Autodesk Fusion 360 part; units mm, degrees
sketch "profile" plane through (0, 0, 0) normal (0, 0, 1) x (1, 0, 0)
  line L0 (0, 0) -> (0, 14)
  line L1 (21.6, 10.2) -> (19.6, 11.8)
  line L2 (19.6, 11.8) -> (21.8, 14)
  line L3 (21.8, 14) -> (25.6, 14)
  line L4 (4, 10.2) -> (6, 11.8)
  line L5 (6, 11.8) -> (3.8, 14)
  line L6 (3.8, 14) -> (0, 14)
  line L7 (4, 4) -> (21.6, 4)
  line L8 (4, 10.2) -> (4, 4)
  line L9 (21.6, 4) -> (21.6, 10.2)
  line L10 (0, 0) -> (25.6, 0)
  line L11 (25.6, 14) -> (25.6, 0)
  dimension "d74" = 3.8
  dimension "d75" = 3.8
  dimension "d76" = 4
  dimension "d80" = 17.6
  dimension "d84" = 4
  dimension "d85" = 14
  dimension "d86" = 14
  dimension "d87" = 3.8
  dimension "d88" = 6
  dimension "d89" = 4
  dimension "d90" = 25.8
  dimension "d117" = 6
  dimension "d118" = 3.8
  dimension "d119" = 1.6
  dimension "d120" = 1.6
extrude "Extrude2" add sketch "profile" along normal blind 130
move_body "Move1" bodies 1 to x (1, 0, 0) y (0, 0, 1) z (0, -1, 0) at (0, 6.5916, 6.5916)
hole "Hole4" at (25.6, -58.4084, 13.5916) direction (-1, 0, 0) diameter 2.529 depth 42 tip angle 180
fillet "Fillet5" radius 2 1 edges at (25.6, -58.4084, 20.5916)
fillet "Fillet6" radius 2 1 edges at (0, -58.4084, 20.5916)
fillet "Fillet7" radius 2 2 edges at (21.8, -58.4084, 20.5916) (3.8, -58.4084, 20.5916)
fillet "Fillet8" radius 1 5 edges at (12.8, 6.5916, 10.5916) (21.6, 6.5916, 13.6916) (20.6, 6.5916, 17.5916) (5, 6.5916, 17.5916) (4, 6.5916, 13.6916)
fillet "Fillet9" radius 1 5 edges at (4, -123.4084, 13.6916) (21.6, -123.4084, 13.6916) (12.8, -123.4084, 10.5916) (5, -123.4084, 17.5916) (20.6, -123.4084, 17.5916)
move_body "Align2" bodies 1 to x (1, 0, 0) y (0, 1, 0) z (0, 0, 1) at (0, 0, -6.5916)
fillet "Fillet10" radius 1 26 edges at (25.6, -123.4084, 6) (25.0142, -123.4084, 13.4142) (23.1142, -123.4084, 14) (21.8631, -123.4084, 13.8478) (20.7628, -123.4084, 12.9628) (19.8084, -123.1155, 12.0084) (19.6, -58.4084, 11.8) (19.8084, 6.2987, 12.0084) (20.7628, 6.5916, 12.9628) (21.8631, 6.5916, 13.8478) (23.1142, 6.5916, 14) (25.0142, 6.5916, 13.4142) (25.6, 6.5916, 6) (0, 6.5916, 6) (0.5858, 6.5916, 13.4142) (2.4858, 6.5916, 14) (3.7369, 6.5916, 13.8478) (4.8372, 6.5916, 12.9628) (5.7916, 6.2987, 12.0084) (6, -58.4084, 11.8) (5.7916, -123.1155, 12.0084) (4.8372, -123.4084, 12.9628) (3.7369, -123.4084, 13.8478) (2.4858, -123.4084, 14) (0.5858, -123.4084, 13.4142) (0, -123.4084, 6)
hole "Hole5" at (12.8, -113.4084, 4) direction (0, 0, -1) diameter 5.5 depth 4 tip angle 180 countersink diameter 10.4 countersink angle 90
hole "Hole6" at (12.8, -3.4084, 4) direction (0, 0, -1) diameter 5.5 depth 15 tip angle 180 countersink diameter 10.4 countersink angle 90
equation "insideheight = 10 mm"
equation "d85 = height"
equation "d86 = height"
equation "height = 14 mm"
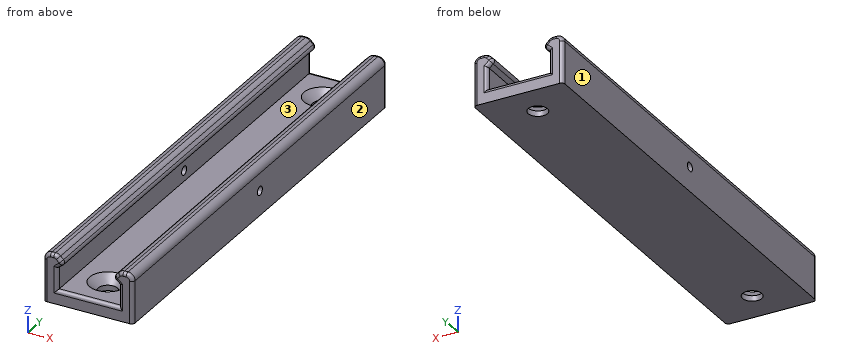
Work out the finished part from the listing and answer in its coordinate system (mm). Face numbers are marked on the shaded views. Coordinates: 2 decimals unless noted, no trailing zeros. Write each loop counter-clockwise with the first axis right and the second up, starting at its lowest first coordinate (ties: lowest second). Pieces come first, ordered by that corner, then holes.
Q1. A cutting plane is placed at B-B, the plane x = 12.8. Give the vertices of the cut face in (y, z), then the cut area to 3 significant figures.
Q2. A cutting plane is placed at C-C, the plane y = -53. Give the vertices of the cut face in (x, z), then the cut area to 3 significant figures.
Q3. Each of these flat-tipped pins is pushed along its axis until it touches: pin 1 Ø9 at (x, y) = (12.8, -113.41) entering from +Z; pin 2 Ø5 at (x, z) = (6.5, 10) entering from -Y. Where does it stop, or does it pass through?
Q4. Determine the mould class of the marked faces 1, 2 and 3 for opening direction X: released by +X, released by -X, zero draft, split by the parting line, or undercut.
Q5. A cutting plane is placed at A-A, the plane z = 7. Give the vertices of the cut face in (x, y), then the cut area to 3 significant figures.
Q6. Find the intervals of material crossed by line 1 (Y direction, x = 2.65, z = 7); line 2 (X direction, y = -63, z = 8); line 3 (Y direction, x = 12.8, z = 0.5), in increasing order.
Findings below:
1. outline: (-123.41, 0) - (-116.16, 0) - (-116.16, 1.55) - (-118.61, 4) - (-122.41, 4) arc R1 ccw to (-123.41, 3) - close; (-110.66, 0) - (-6.16, 0) - (-6.16, 1.55) - (-8.61, 4) - (-108.21, 4) - (-110.66, 1.55) - close; (-0.66, 0) - (6.59, 0) - (6.59, 3) arc R1 ccw to (5.59, 4) - (1.79, 4) - (-0.66, 1.55) - close
1. area: 464 mm2
2. outline: (0, 0) - (25.6, 0) - (25.6, 12) arc R2 ccw to (23.6, 14) - (22.63, 14) arc R2 ccw to (21.21, 13.41) - (20.39, 12.59) arc R1 ccw to (20.47, 11.1) - (21.6, 10.2) - (21.6, 4) - (4, 4) - (4, 10.2) - (5.13, 11.1) arc R1 ccw to (5.21, 12.59) - (4.39, 13.41) arc R2 ccw to (2.97, 14) - (2, 14) arc R2 ccw to (0, 12) - close
2. area: 187 mm2
3. pin 1: stops at z = 3.3
3. pin 2: stops at y = -123.38
4. face 1: released by -X
4. face 2: released by +X
4. face 3: undercut
5. outline: (0, -122.41) arc R1 ccw to (1, -123.41) - (3, -123.41) arc R1 ccw to (4, -122.41) - (4, -59.67) - (0, -59.67) - close; (0, -57.14) - (4, -57.14) - (4, 5.59) arc R1 ccw to (3, 6.59) - (1, 6.59) arc R1 ccw to (0, 5.59) - close; (21.6, -122.41) arc R1 ccw to (22.6, -123.41) - (24.6, -123.41) arc R1 ccw to (25.6, -122.41) - (25.6, -59.67) - (21.6, -59.67) - close; (21.6, -57.14) - (25.6, -57.14) - (25.6, 5.59) arc R1 ccw to (24.6, 6.59) - (22.6, 6.59) arc R1 ccw to (21.6, 5.59) - close
5. area: 1,020 mm2
6. line 1: y = -123.41 to -59.67, -57.14 to 6.59
6. line 2: x = 0 to 4, 21.6 to 25.6
6. line 3: y = -123.41 to -116.16, -110.66 to -6.16, -0.66 to 6.59
